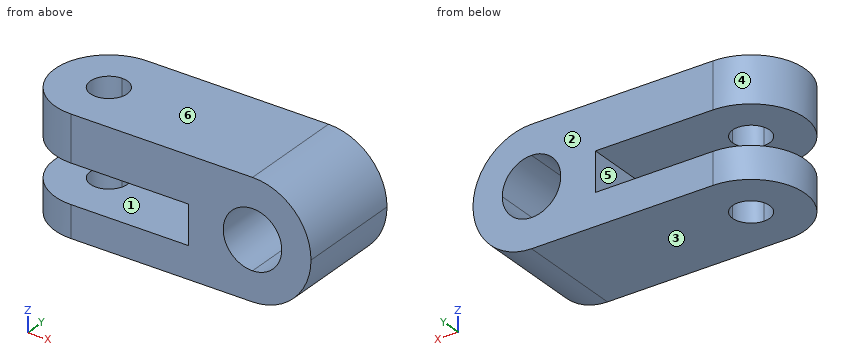
from build123d import *

# Parameters (mm, degrees)
F1_DEPTH  = 40.64
F3_DEPTH  = 44.196
F4_W      = 44.45
F4_H      = 14.732
F5_DEPTH  = 40.641
F6_W      = 20.32
F6_H      = 14.732
F7_DEPTH  = 40.641
F9_DEPTH  = 44.197
F11_DEPTH = 40.641


with BuildPart() as f1:
    # F0 (on Front) → F1 (new body)
    with BuildSketch(Plane.XZ):
        with BuildLine():
            Line((68.58, 0), (0, 0))
            Line((0, 0), (0, -44.196))
            Line((0, -44.196), (68.58, -44.196))
            ThreePointArc((68.58, -44.196), (46.482, -22.098), (68.58, 0))
        make_face()
        with BuildLine():
            ThreePointArc((90.678, -22.098), (84.2056456507, -6.4723543493), (68.58, 0))
            Line((68.58, 0), (68.58, -44.196))
            ThreePointArc((68.58, -44.196), (84.2056456507, -37.7236456507), (90.678, -22.098))
        make_face()
        with BuildLine():
            Line((68.58, -44.196), (68.58, 0))
            ThreePointArc((68.58, 0), (46.482, -22.098), (68.58, -44.196))
        make_face()
    extrude(amount=F1_DEPTH)

    # F2 (on face) → F3 (join)
    with BuildSketch(Plane.XY):
        with BuildLine():
            Line((0, -40.64), (0, 0))
            ThreePointArc((0, 0), (-20.32, -20.32), (0, -40.64))
        make_face()
    extrude(amount=-F3_DEPTH)

    # F4 (on face) → F5 (cut, through all)
    with BuildSketch(Plane.XZ.offset(40.64)):
        with Locations((22.225, -24.7622483637)):
            Rectangle(F4_W, F4_H)
    extrude(amount=-F5_DEPTH, mode=Mode.SUBTRACT)

    # F6 (on face) → F7 (cut, through all)
    with BuildSketch(Plane.XZ.offset(40.64)):
        with Locations((-10.16, -24.7622483637)):
            Rectangle(F6_W, F6_H)
    extrude(amount=-F7_DEPTH, mode=Mode.SUBTRACT)

    # F8 (on face) → F9 (cut, through all)
    with BuildSketch(Plane.XY):
        with BuildLine():
            ThreePointArc((0, -13.335), (-6.985, -20.32), (0, -27.305))
            Line((0, -27.305), (0, -13.335))
        make_face()
        with BuildLine():
            Line((0, -13.335), (0, -27.305))
            ThreePointArc((0, -27.305), (4.9391408666, -25.2591408666), (6.985, -20.32))
            ThreePointArc((6.985, -20.32), (4.9391408666, -15.3808591334), (0, -13.335))
        make_face()
    extrude(amount=-F9_DEPTH, mode=Mode.SUBTRACT)

    # F10 (on face) → F11 (cut, through all)
    with BuildSketch(Plane.XZ.offset(40.64)):
        with BuildLine():
            ThreePointArc((79.629, -22.098), (76.3928228253, -14.2851771747), (68.58, -11.049))
            Line((68.58, -11.049), (68.58, -33.147))
            ThreePointArc((68.58, -33.147), (76.3928228253, -29.9108228253), (79.629, -22.098))
        make_face()
        with BuildLine():
            Line((68.58, -33.147), (68.58, -11.049))
            ThreePointArc((68.58, -11.049), (57.531, -22.098), (68.58, -33.147))
        make_face()
    extrude(amount=-F11_DEPTH, mode=Mode.SUBTRACT)


solid = f1.part
The listing builds one solid part. Answer for the finished solid, in the listing's coordinates (mm). Face numbers are marked on the shaded views. A direction names the side the tool comes from. Give positions to 0.01 mm unless a question says otherwise; leave off trailing zeros. Loops run counter-clockwise (first coordinate to the right, second up) from the corner with the lowest first, then second, coordinate; pieces in that order, holes last. Notation, with made-up numbers: M -16.75,-21 L 34.25,-21 A13 cw 34.25,-3 Z; hole C -10.75,0 d1. An arc over 180 degrees is marked long. Answer as CSV lines item,"result".
Item 1: Which of the six approach directions +Z, -Z, +X, -X, +Y, -Y give full straight-line access (tool end or side, diameter ignored) to the marked faces 1 and 2?
Values follow:
face 1,"-X, +Y, -Y"
face 2,"+Z, -Z, +X, -X, +Y"
Item 2: The part is cut by section C-C (z = -36). Give the vertices of the cut face in (x, y) (3 decimals).
Values follow:
outline,"M 0,-40.64 L 85.757,-40.64 L 85.757,0 L 0,0 A20.32 ccw Z; hole C 0,-20.32 d13.97"
Item 3: The part is cut by section A-A (x = 20.5). Give the vertices of the cut face in (y, z).
Values follow:
outline,"M -40.64,-44.2 L 0,-44.2 L 0,-32.13 L -40.64,-32.13 Z; M -40.64,-17.4 L 0,-17.4 L 0,0 L -40.64,0 Z"
Item 4: The part is cut by section B-B (z = -30). Give the vertices of the cut face in (x, y), and give its area (3 significant figures).
Values follow:
outline,"M 44.45,-40.64 L 60.86,-40.64 L 60.86,0 L 44.45,0 Z; M 76.3,-40.64 L 89.22,-40.64 L 89.22,0 L 76.3,0 Z"
area,"1,190 mm^2"
Item 5: Given pin 1 Ø1.5 at (y, z) = (-16, -15) entering from +X; pin 2 Ø10 at (y, z) = (-4.5, -37) entering from +X; pin 3 Ø4.5 at (y, z) = (-19.5, -28.5) entering from -X; pin 4 Ø6 at (x, z) = (30.5, -26.5) entering from +Y, each flat-ended and moving along its own axis, determine where each tip first touches the part or whether it passes through.
Values follow:
pin 1,"stops at x = 89.75"
pin 2,"stops at x = 88.34"
pin 3,"stops at x = 44.45"
pin 4,"passes through"
Item 6: The mould has two halves that part along Z. Classify the marked faces 3, 4, 5 and 6: released by +Z, released by -Z, zero draft, split by the parting line, or undercut.
Values follow:
face 3,"released by -Z"
face 4,"zero draft"
face 5,"undercut"
face 6,"released by +Z"
Item 7: The part is cut by section D-D (y = -38). Give the vertices of the cut face in (x, z).
Values follow:
outline,"M -10.02,-44.2 L 68.58,-44.2 A22.1 ccw 68.58,0 L -10.02,0 L -10.02,-17.4 L 44.45,-17.4 L 44.45,-32.13 L -10.02,-32.13 Z; hole C 68.58,-22.1 d22.1"
Item 8: Straight lines are drawn through the part: line 1 along X through (y, z) = (-35.5, -22); line 2 along Z through (x, y) = (-2.5, -38); line 3 along X through (y, z) = (-14, -26). For each, find the intervals that lie inside material, in ascending order. Write a range as [from, to].
Values follow:
line 1,"x = [44.45, 57.53], [79.63, 90.68]"
line 2,"z = [-44.2, -32.13], [-17.4, 0]"
line 3,"x = [44.45, 58.24], [78.92, 90.33]"
